Design review of the part built by this model. Coordinates are the model's own, in mm. A direction names the side the tool comes from. Give positions to 0.01 mm unless a question says otherwise; leave off trailing zeros. Order: outer loops, then holes, each group sorted by start corner. A loop starts at its lowest first (then second) coordinate and runs counter-clockwise, first axis right, second up. Notation, with made-up numbers: M 83.5,17.25 L 131.5,17.25 A24 ccw 131.5,43.25 Z; hole C -37.5,83.25 d4. An arc over 180 degrees is marked long. Answer as a JSON object with one key per item and string values.
from build123d import *

# Parameters (mm, degrees)
CROQUIS1_R              = 1.7
SALIENTE_EXTRUIR1_DEPTH = 3.75
CROQUIS2_R              = 3.15
SALIENTE_EXTRUIR2_DEPTH = 0.63
SALIENTE_EXTRUIR3_DEPTH = 2.2
CROQUIS4_R              = 2.365
SALIENTE_EXTRUIR4_DEPTH = 28.6
CROQUIS5_R              = 0.95
SALIENTE_EXTRUIR5_DEPTH = 2.2
CROQUIS6_R              = 1.25
CORTAR_EXTRUIR1_DEPTH   = 0.5
CROQUIS7_R              = 2.5
CORTAR_EXTRUIR2_DEPTH   = 1.8


with BuildPart() as part:
    # Croquis1 → Saliente-Extruir1 (new body)
    with BuildSketch(Plane.XY):
        with BuildLine():
            Line((0, 3.15), (47.88, 3.15))
            ThreePointArc((47.88, 3.15), (51.03, 0), (47.88, -3.15))
            Line((47.88, -3.15), (0, -3.15))
            ThreePointArc((0, -3.15), (-3.15, 0), (0, 3.15))
        make_face()
        Circle(CROQUIS1_R, mode=Mode.SUBTRACT)
    extrude(amount=SALIENTE_EXTRUIR1_DEPTH)

    # Croquis2 → Saliente-Extruir2 (add)
    with BuildSketch(Plane.XY.offset(3.75)):
        with Locations(Location((47.88, 0, 0), (0, 0, 90))):
            Circle(CROQUIS2_R)
    extrude(amount=SALIENTE_EXTRUIR2_DEPTH)

    # Croquis3 → Saliente-Extruir3 (add)
    with BuildSketch(Plane.XY.offset(4.38)):
        with BuildLine():
            Line((44.73, 15.75), (44.73, 0))
            ThreePointArc((44.73, 0), (47.88, -3.15), (51.03, 0))
            Line((51.03, 0), (51.03, 15.75))
            ThreePointArc((51.03, 15.75), (47.88, 18.9), (44.73, 15.75))
        make_face()
    extrude(amount=SALIENTE_EXTRUIR3_DEPTH)

    # Croquis4 → Saliente-Extruir4 (add)
    with BuildSketch(Plane.XY.offset(6.58)):
        with Locations((47.88, 15.75)):
            Circle(CROQUIS4_R)
    extrude(amount=SALIENTE_EXTRUIR4_DEPTH)

    # Croquis5 → Saliente-Extruir5 (add)
    with BuildSketch(Plane.XY.offset(35.18)):
        with BuildLine():
            Line((44.73, 15.75), (44.73, 0))
            ThreePointArc((44.73, 0), (47.88, -3.15), (51.03, 0))
            Line((51.03, 0), (51.03, 15.75))
            ThreePointArc((51.03, 15.75), (47.88, 18.9), (44.73, 15.75))
        make_face()
        with Locations((47.88, 0)):
            Circle(CROQUIS5_R, mode=Mode.SUBTRACT)
    extrude(amount=SALIENTE_EXTRUIR5_DEPTH)

    # Croquis6 → Cortar-Extruir1 (cut)
    with BuildSketch(Plane(origin=(0, 0, 35.18), x_dir=(-1, 0, 0), z_dir=(0, 0, -1))):
        with Locations((-47.88, 0)):
            Circle(CROQUIS6_R)
    extrude(amount=-CORTAR_EXTRUIR1_DEPTH, mode=Mode.SUBTRACT)

    # Croquis7 → Cortar-Extruir2 (cut)
    with BuildSketch(Plane(origin=(0, 0, 0), x_dir=(-1, 0, 0), z_dir=(0, 0, -1))):
        Circle(CROQUIS7_R)
    extrude(amount=-CORTAR_EXTRUIR2_DEPTH, mode=Mode.SUBTRACT)


solid = part.part
(1) Tool access review of faces 1 (the flat face through (-2, -1, 1.8)), 2 (the flat face through (44.73, 8, 5)), 3 (the cylindrical face through (46.69, 0.38, 35.43)): name each direction out of +Z, -Z, +X, -X, +Y, -Y from which nothing blocks a thin tool from reaching the whole face with its end or side.
Checked values:
{"face 1": "-Z", "face 2": "+Z, -X, +Y, -Y", "face 3": "none"}
(2) We need section A-A (y = 11). Write out the cut boundary in (x, z).
Checked values:
{"outline": "M 44.73,4.38 L 51.03,4.38 L 51.03,6.58 L 44.73,6.58 Z; M 44.73,35.18 L 51.03,35.18 L 51.03,37.38 L 44.73,37.38 Z"}
(3) Draft analysis for pull direction Y (two halves, no side actions). For faces 4 (the flat face through (23, 0, 3.75)), 5 (the cylindrical face through (50.955, -0.683, 3.244)), 6 (the cylindrical face through (-0.37, -1.66, 2.76)), state which applies: +Y half, -Y half, draft (parallel to the pull), parting line (faces both ways), or undercut.
Checked values:
{"face 4": "draft", "face 5": "parting line", "face 6": "undercut"}
(4) To check wall thickness, follow L1, parallel to Y at x = 0, z = 2.5; L2, parallel to Y at x = 47.88, z = 36.35; L3, parallel to X at y = 2.25, z = 4.5. State the ranges of each line that lie inside material, in increasing order. Write a range as from..to.
Checked values:
{"L1": "y = -3.15..-1.7, 1.7..3.15", "L2": "y = -3.15..-0.95, 0.95..18.9", "L3": "x = 44.73..51.03"}
(5) We need section B-B (x = 38). Write out the cut boundary in (y, z).
Checked values:
{"outline": "M -3.15,0 L 3.15,0 L 3.15,3.75 L -3.15,3.75 Z"}
(6) We need section C-C (z = 34). Write out the cut boundary in (x, y) (3 decimals), plus the area to 3 significant figures.
Checked values:
{"outline": "C 47.88,15.75 d4.73", "area": "17.6 mm^2"}
(7) Insertion check: pin 1 (1.2 mm diameter, centred on x = 48, y = 0.5, fed in from -Z); pin 2 (5 mm diameter, centred on x = 10, y = -1.5, fed in from +Z); pin 3 (2.5 mm diameter, centred on y = 8.5, z = 5.5, fed in from -X); pin 4 (4 mm diameter, centred on x = 17, z = 2, fed in from +Y). Each pin has a flat end and moves straight along its axis. Give the tip position at first contact, or say it passes through.
Checked values:
{"pin 1": "stops at z = 0", "pin 2": "stops at z = 3.75", "pin 3": "stops at x = 44.73", "pin 4": "stops at y = 3.15"}
